Work out the finished part from the listing and answer in its coordinate system (mm). Face numbers are marked on the shaded views. A direction names the side the tool comes from. Coordinates: 2 decimals unless noted, no trailing zeros. Order: outer loops, then holes, each group sorted by start corner. A loop starts at its lowest first (then second) coordinate and runs counter-clockwise, first axis right, second up.
Autodesk Inventor part; units mm, degrees
ref_plane "YZ Plane" through (0, 0, 0) normal (1, 0, 0) x (0, 1, 0)
ref_plane "XZ Plane" through (0, 0, 0) normal (0, 1, 0) x (-1, 0, 0)
ref_plane "XY Plane" through (0, 0, 0) normal (0, 0, 1) x (1, 0, 0)
sketch "スケッチ1" plane through (0, 0, 0) normal (1, 0, 0) x (0, 1, 0)
  line L0 (7.8325, 11.4458) -> (-8.7675, 11.4458)
  line L1 (-8.7675, 11.4458) -> (-8.7675, -38.5542)
  line L2 (-8.7675, -38.5542) -> (7.8325, -38.5542)
  line L3 (7.8325, -38.5542) -> (7.8325, 11.4458)
  circle A0 centre (-0.4675, 6.9458) radius 2.5
  line L4 (7.8325, 11.4458) -> (-8.7675, 11.4458)
  line L5 (-8.7675, 11.4458) -> (-8.7675, -38.5542)
  line L6 (-8.7675, -38.5542) -> (7.8325, -38.5542)
  line L7 (7.8325, -38.5542) -> (7.8325, 11.4458)
  circle A1 centre (-0.4675, 6.9458) radius 2.5
  point P0 (0, 0)
  point P1 (0, 0)
  point P2 (0, 0)
  dimension "d0" = 16.6
  dimension "d1" = 5
  dimension "d2" = 8.3
  dimension "d3" = 8.3
  dimension "d4" = 4.5
  dimension "d5" = 2
  dimension "d6" = 50
  dimension "d7" = 16.6
  dimension "d8" = 5
  dimension "d9" = 8.3
  dimension "d10" = 8.3
  dimension "d11" = 4.5
  dimension "d12" = 2
  dimension "d13" = 50
extrude "押し出し1" add sketch "スケッチ1" along normal blind 3
sketch "スケッチ2" plane through (3, 0, 0) normal (1, 0, 0) x (0, 0, -1)
  line L0 (-11.4458, -8.7675) -> (38.5542, -8.7675)
  line L1 (38.5542, 7.8325) -> (-11.4458, 7.8325)
  line L2 (38.5542, -8.7675) -> (28.5542, -8.7675)
  line L3 (28.5542, -8.7675) -> (28.5542, 7.8325)
  line L4 (28.5542, 7.8325) -> (38.5542, 7.8325)
  line L5 (38.5542, 7.8325) -> (38.5542, -8.7675)
  point P0 (0, 0)
  dimension "d16" = 10
extrude "押し出し2" add sketch "スケッチ2" along normal blind 25
sketch "スケッチ3" plane through (0, 0, 0) normal (-1, 0, 0) x (0, 0, 1)
  line L0 (-28.5542, 7.8325) -> (11.4458, 7.8325)
  line L1 (-38.5542, -8.7675) -> (-38.5542, 7.8325)
  line L2 (11.4458, 7.8325) -> (-38.5542, 7.8325)
  line L3 (-38.5542, 7.8325) -> (-38.5542, -8.7675)
  line L4 (-38.5542, -8.7675) -> (11.4458, -8.7675)
  line L5 (11.4458, -8.7675) -> (11.4458, 7.8325)
  circle A0 centre (6.9458, -0.4675) radius 2.5
  circle A1 centre (6.9458, -0.4675) radius 1.5
  point P0 (0, 0)
  dimension "d19" = 3
extrude "押し出し3" add sketch "スケッチ3" along normal blind 1 contours L0 L5 L4 L1 L2 | A0
sketch "スケッチ4" plane through (28, 0, 0) normal (1, 0, 0) x (0, 0, -1)
  circle A0 centre (33.5542, -5.7675) radius 1.5
  circle A1 centre (33.5542, 4.8325) radius 1.5
  line L0 (28.5542, -8.7675) -> (38.5542, -8.7675)
  line L1 (38.5542, 7.8325) -> (28.5542, 7.8325)
  line L2 (28.5542, 7.8325) -> (28.5542, -8.7675)
  point P0 (0, 0)
  dimension "d22" = 3
  dimension "d23" = 3
  dimension "d24" = 3
  dimension "d25" = 3
  dimension "d26" = 5
  dimension "d27" = 5
extrude "押し出し4" cut sketch "スケッチ4" against normal blind 100
properties part number "armpart4"
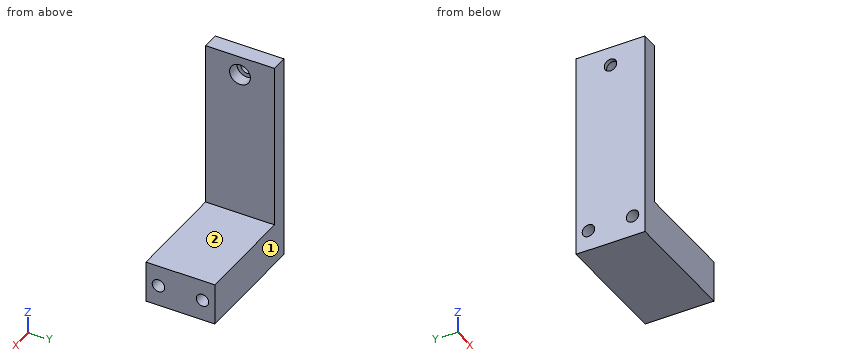
1. For the marked faces 1 and 2, determine the directions among +Z, -Z, +X, -X, +Y, -Y from which every point of the face is accessible in a straight line to the end or side of a thin tool.
2. The part is cut by section C-C (z = 6). Determine the outline of the cut face in (x, y), plus the area to 3 significant figures.
3. The part is cut by section D-D (x = 6.5). Determine the outline of the cut face in (y, z), plus the area to 3 significant figures.
4. Consider probe 1 along X at (y, z) = (0.75, 5); probe 2 along X at (y, z) = (-5.25, 7); probe 3 along Z at (x, y) = (4.25, 6.75). Determine where each line is inside the solid, lowest interval first.
5. The part is cut by section A-A (y = -5). Determine the outline of the cut face in (x, z), plus the area to 3 significant figures.
6. The part is cut by section B-B (z = -33). Determine the outline of the cut face in (x, y).
7. Flat-ended cylindrical pins translate along their axes: pin 1 (2 mm diameter, centred on y = 2.5, z = -20, fed in from +X); pin 2 (2.5 mm diameter, centred on y = -5.77, z = -33.55, fed in from +X); pin 3 (5 mm diameter, centred on x = 16.5, y = 3.5, fed in from +Z). Find the tip coordinate at first contact, or state that the pin passes through.
Worked out:
1. face 1: +Z, -Z, +X, -X, +Y
1. face 2: +Z, +X, +Y, -Y
2. outline: (-1, -8.77) - (3, -8.77) - (3, -2.78) - (0, -2.78) - (0, -1.63) - (-1, -1.63) - close; (-1, 0.7) - (0, 0.7) - (0, 1.85) - (3, 1.85) - (3, 7.83) - (-1, 7.83) - close
2. area: 50.2 mm2
3. outline: (-8.77, -38.55) - (7.83, -38.55) - (7.83, -28.55) - (-8.77, -28.55) - close; hole circle Ø3 at (-5.77, -33.55); hole circle Ø3 at (4.83, -33.55)
3. area: 152 mm2
4. probe 1: x = -1 to 0
4. probe 2: x = -1 to 3
4. probe 3: z = -38.55 to -28.55
5. outline: (-1, -38.55) - (28, -38.55) - (28, -34.84) - (-1, -34.84) - close; (-1, -32.27) - (28, -32.27) - (28, -28.55) - (3, -28.55) - (3, 11.45) - (-1, 11.45) - close
5. area: 375 mm2
6. outline: (-1, -8.77) - (28, -8.77) - (28, -7.16) - (-1, -7.16) - close; (-1, -4.37) - (28, -4.37) - (28, 3.44) - (-1, 3.44) - close; (-1, 6.23) - (28, 6.23) - (28, 7.83) - (-1, 7.83) - close
7. pin 1: stops at x = 3
7. pin 2: passes through
7. pin 3: stops at z = -28.55
